The drawing under review shows one solid part. Ordinate dimensions are in mm from its lowest x, y, z. A direction names the side the tool comes from. Coordinates: 2 decimals unless noted, no trailing zeros. Order: outer loops, then holes, each group sorted by start corner. A loop starts at its lowest first (then second) coordinate and runs counter-clockwise, first axis right, second up. Notation, with made-up numbers: (50.25, -5.75) - (83.25, -5.75) arc R17 cw to (83.25, 10.25) - close; hole circle Ø4 at (-16.75, 46). An arc over 180 degrees is marked (long way). Answer in a Markdown table with one row per item.
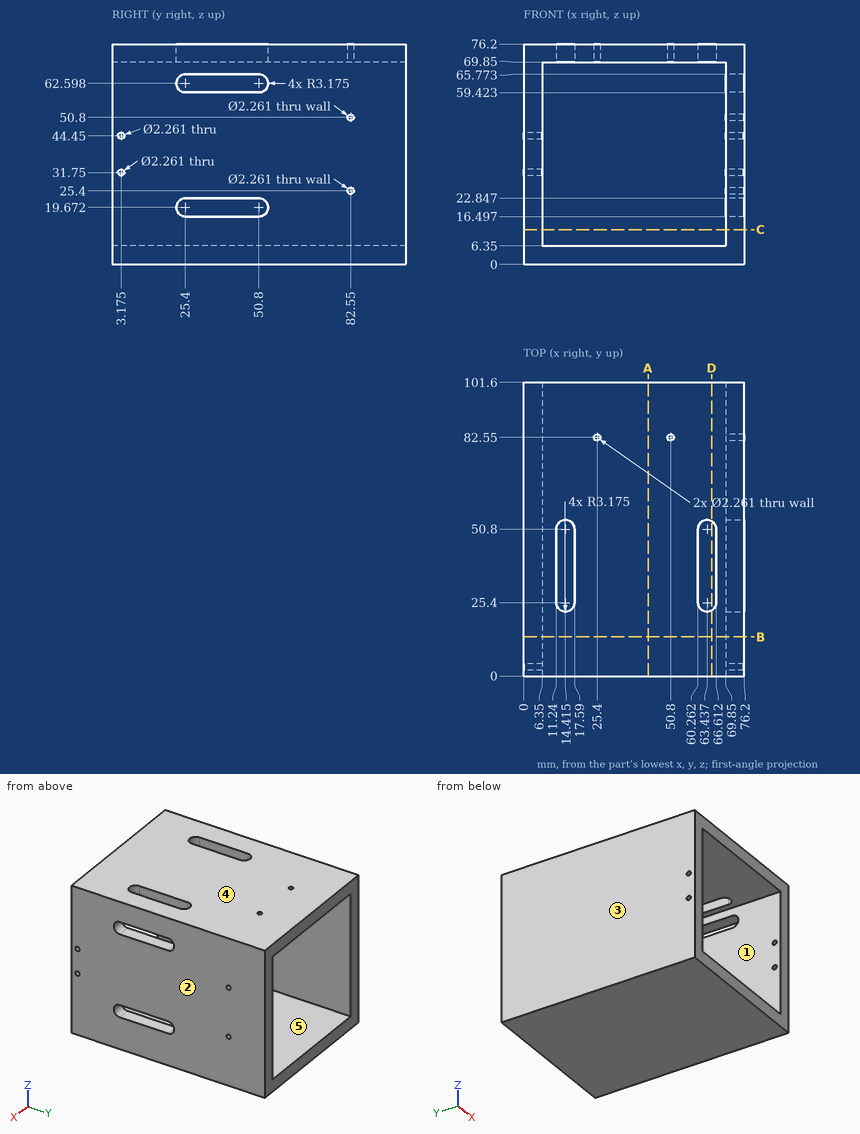
Item 1: We need section A-A, the plane x = 43. Write out the cut boundary in (y, z).
Check values:
| item | result |
|---|---|
| outline | (0, 0) - (101.6, 0) - (101.6, 6.35) - (0, 6.35) - close; (0, 69.85) - (101.6, 69.85) - (101.6, 76.2) - (0, 76.2) - close |
Item 2: To check wall thickness, follow line 1 (X direction, y = 82.55, z = 73.5); line 2 (X direction, y = 39.5, z = 70); line 3 (Z direction, x = 29, y = 85). State the ranges of each line that lie inside material, in increasing order. Write a range as from..to.
Check values:
| item | result |
|---|---|
| line 1 | 0..24.27, 26.53..49.67, 51.93..76.2 |
| line 2 | 0..11.24, 17.59..60.26, 66.61..76.2 |
| line 3 | 0..6.35, 69.85..76.2 |
Item 3: Mouldability with a two-part tool opening along X and no side actions: class the marked faces 1, 2 and 3 as +X half, -X half, draft (parallel to the pull), parting line (faces both ways), or undercut.
Check values:
| item | result |
|---|---|
| face 1 | undercut |
| face 2 | +X half |
| face 3 | -X half |
Item 4: We need section B-B, the plane y = 13.5. Write out the cut boundary in (x, z).
Check values:
| item | result |
|---|---|
| outline | (0, 0) - (76.2, 0) - (76.2, 76.2) - (0, 76.2) - close; hole (6.35, 6.35) - (69.85, 6.35) - (69.85, 69.85) - (6.35, 69.85) - close |
Item 5: We need section C-C, the plane z = 12. Write out the cut boundary in (x, y), then the cut area to 3 significant figures.
Check values:
| item | result |
|---|---|
| outline | (0, 0) - (6.35, 0) - (6.35, 101.6) - (0, 101.6) - close; (69.85, 0) - (76.2, 0) - (76.2, 101.6) - (69.85, 101.6) - close |
| area | 1,290 mm^2 |
Item 6: Clearance check with a flat-ended pin moving along its axis: pin 1 Ø2 at (y, z) = (82.55, 50.8) entering from +X. State where the tip first meets the part, or that it passes through.
Check values:
| item | result |
|---|---|
| pin 1 | x = 6.35 |
Item 7: Tool access review of the marked faces 4 and 5: name each direction out of +Z, -Z, +X, -X, +Y, -Y from which nothing blocks a thin tool from reaching the whole face with its end or side.
Check values:
| item | result |
|---|---|
| face 4 | +Z, +X, -X, +Y, -Y |
| face 5 | +Y, -Y |
Item 8: We need section D-D, the plane x = 65. Write out the cut boundary in (y, z).
Check values:
| item | result |
|---|---|
| outline | (0, 0) - (101.6, 0) - (101.6, 6.35) - (0, 6.35) - close; (0, 69.85) - (22.64, 69.85) - (22.64, 76.2) - (0, 76.2) - close; (53.56, 69.85) - (101.6, 69.85) - (101.6, 76.2) - (53.56, 76.2) - close |
